```python
from build123d import *

# Parameters (mm, degrees)
SKETCH1_R           = 12.7
BOSS_EXTRUDE1_DEPTH = 5.08
SKETCH2_R           = 0.9906
CUT_EXTRUDE1_DEPTH  = 19.66511184
SKETCH3_R           = 2
CUT_EXTRUDE2_DEPTH  = 19.66511184
SKETCH4_R           = 2
BOSS_EXTRUDE2_DEPTH = 5.08


with BuildPart() as part:
    # Sketch1 → Boss-Extrude1 (new body)
    with BuildSketch(Plane.XY):
        Circle(SKETCH1_R)
    extrude(amount=BOSS_EXTRUDE1_DEPTH)

    # Sketch2 → Cut-Extrude1 (cut, through all)
    with BuildSketch(Plane.XY.offset(5.08)):
        Circle(SKETCH2_R)
    extrude(amount=-CUT_EXTRUDE1_DEPTH, mode=Mode.SUBTRACT)

    # Sketch3 → Cut-Extrude2 (cut, through all)
    with BuildSketch(Plane.XY.offset(5.08)):
        with Locations((0, 9.652)):
            Circle(SKETCH3_R)
    extrude(amount=-CUT_EXTRUDE2_DEPTH, mode=Mode.SUBTRACT)

    # Sketch4 → Boss-Extrude2 (add)
    with BuildSketch(Plane.XY.offset(5.08)):
        with Locations((0, -8.909221011)):
            Circle(SKETCH4_R)
    extrude(amount=BOSS_EXTRUDE2_DEPTH)


solid = part.part
```
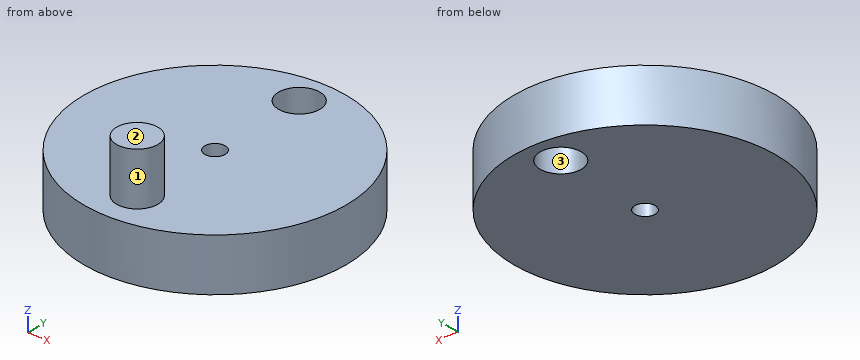
Verification items for the finished model (mm, model axes). Face numbers are marked on the shaded views. Round coordinates to 2 decimals unless told otherwise and drop trailing zeros. Order: outer loops, then holes, each group sorted by start corner. A loop starts at its lowest first (then second) coordinate and runs counter-clockwise, first axis right, second up.
1) Cross-section at B-B, the plane x = 0. Record the cut outline in (y, z), plus the area to 3 significant figures.
Geometry says:
outline: (-12.7, 0) - (-0.99, 0) - (-0.99, 5.08) - (-6.91, 5.08) - (-6.91, 10.16) - (-10.91, 10.16) - (-10.91, 5.08) - (-12.7, 5.08) - close; (0.99, 0) - (7.65, 0) - (7.65, 5.08) - (0.99, 5.08) - close; (11.65, 0) - (12.7, 0) - (12.7, 5.08) - (11.65, 5.08) - close
area: 119 mm2
2) Cross-section at D-D, the plane z = 2. Record the cut outline in (x, y), plus the area to 3 significant figures.
Geometry says:
outline: circle Ø25.4 at (0, 0); hole circle Ø4 at (0, 9.65); hole circle Ø1.98 at (0, 0)
area: 491 mm2
3) Cross-section at C-C, the plane y = -8. Record the cut outline in (x, z), plus the area to 3 significant figures.
Geometry says:
outline: (-9.86, 0) - (9.86, 0) - (9.86, 5.08) - (1.78, 5.08) - (1.78, 10.16) - (-1.78, 10.16) - (-1.78, 5.08) - (-9.86, 5.08) - close
area: 118 mm2
4) Depth check by flat-ended pin: pin 1 (1 mm diameter, centred on y = 10, z = 3, fed in from -X); pin 2 (6 mm diameter, centred on y = 4, z = 6.5, fed in from +X); pin 3 (6 mm diameter, centred on y = 6, z = 3, fed in from -X). Enter the tip coordinate at first touch or a pass-through.
Geometry says:
pin 1: stops at x = -8.43
pin 2: stops at x = 12.63
pin 3: stops at x = -12.34
5) Cross-section at A-A, the plane y = 0. Record the cut outline in (x, z), plus the area to 3 significant figures.
Geometry says:
outline: (-12.7, 0) - (-0.99, 0) - (-0.99, 5.08) - (-12.7, 5.08) - close; (0.99, 0) - (12.7, 0) - (12.7, 5.08) - (0.99, 5.08) - close
area: 119 mm2
6) Material ranges on line 1 (Y direction, x = 0, z = 3.5); line 2 (Z direction, x = 1.75, y = -5.5); line 3 (X direction, y = 8.5, z = 4.75), recorded low to high.
Geometry says:
line 1: y = -12.7 to -0.99, 0.99 to 7.65, 11.65 to 12.7
line 2: z = 0 to 5.08
line 3: x = -9.44 to -1.63, 1.63 to 9.44
7) Draft check along Y on the marked faces 1, 2 and 3. Enter one of: +Y half, -Y half, draft (parallel to the pull), parting line (faces both ways), or undercut.
Geometry says:
face 1: parting line
face 2: draft
face 3: undercut
